Verification items for the finished model (mm, model axes). A direction names the side the tool comes from. Coordinates: 2 decimals unless noted, no trailing zeros. Write each loop counter-clockwise with the first axis right and the second up, starting at its lowest first coordinate (ties: lowest second). Pieces come first, ordered by that corner, then holes.
```python
from build123d import *

# Parameters (mm, degrees)
CUT_EXTRUDE1_REACH      = 26.41
CUT_EXTRUDE1_END_RADIUS = 1.524
SKETCH2_W               = 0.508
SKETCH2_H               = 0.889
CIRPATTERN1_COUNT       = 16
SKETCH3_R               = 3.556
SKETCH3_R_2             = 1.524
BOSS_EXTRUDE1_DEPTH     = 6.35
BOSS_EXTRUDE2_START     = 6.35
SKETCH4_R               = 19.05
SKETCH4_R_2             = 1.524
BOSS_EXTRUDE2_DEPTH     = 6.35
CUT_EXTRUDE2_REACH      = 51.396
SKETCH11_R              = 1.63195
CIRPATTERN2_COUNT       = 6
CHAMFER1_SIZE           = 3.048
CHAMFER1_SIZE2          = 5.279290861
SKETCH13_R              = 11.43
SKETCH13_R_2            = 6.54812
BOSS_EXTRUDE4_DEPTH     = 12.7
FILLET4_R               = 0.254
CHAMFER2_SIZE           = 0.851662
CHAMFER2_SIZE2          = 0.83947


with BuildPart() as part:
    # Sketch1 → Revolve2 (revolve)
    with BuildSketch(Plane.XY, mode=Mode.PRIVATE) as revolve2_sk:
        with BuildLine():
            Line((-1.524, 23.078774136), (-3.556, 23.078774136))
            Line((-3.556, 23.078774136), (-3.556, -2.067225864))
            ThreePointArc((-3.556, -2.067225864), (-2.514471714, -4.581697578), (0, -5.623225864))
            Line((0, -5.623225864), (0, -1.606607061))
            ThreePointArc((0, -1.606607061), (-0.720373994, -1.97463996), (-1.524, -2.067225864))
            Line((-1.524, -2.067225864), (-1.524, 23.078774136))
        make_face()
    revolve(revolve2_sk.sketch.rotate(Axis((0, 8.215698649, 0), (0, -1, 0)), 270), axis=Axis((0, 8.215698649, 0), (0, -1, 0)))

    # Cut-Extrude1: up to this cylinder (the profile starts outside it)
    cut_extrude1_end = Plane(origin=(0, -0.733726, 0), z_dir=(0, 1, 0)) * Cylinder(CUT_EXTRUDE1_END_RADIUS, 56.868, mode=Mode.PRIVATE)
    # Sketch2 → Cut-Extrude1 (cut, up to the surface)
    with BuildSketch(Plane.ZY.offset(3.556), mode=Mode.PRIVATE) as cut_extrude1_sk1:
        with Locations((0.000240101, -0.733725864)):
            Rectangle(SKETCH2_W, SKETCH2_H)
    cut_extrude1_tool1 = extrude(cut_extrude1_sk1.sketch, amount=-CUT_EXTRUDE1_REACH, mode=Mode.PRIVATE) - cut_extrude1_end
    cut_extrude1 = cut_extrude1_tool1.solids().sort_by_distance((-3.556, -0.733726, 0.00024))[0]
    add(cut_extrude1, mode=Mode.SUBTRACT)

    # CirPattern1: Cut-Extrude1 ×16 about axis
    cirpattern1_axis = Axis((0, 0, 0), (0, 1, 0))
    for i in range(1, CIRPATTERN1_COUNT):
        add(cut_extrude1.rotate(cirpattern1_axis, i * 360 / CIRPATTERN1_COUNT), mode=Mode.SUBTRACT)

    # Sketch3 → Boss-Extrude1 (add)
    with BuildSketch(Plane(origin=(0, 23.078774136, 0), x_dir=(-1, 0, 0), z_dir=(0, -1, 0))):
        with Locations(Location((0, 0, 0), (0, 0, 270))):
            Circle(SKETCH3_R)
        with Locations(Location((0, 0, 0), (0, 0, 270))):
            Circle(SKETCH3_R_2, mode=Mode.SUBTRACT)
    extrude(amount=-BOSS_EXTRUDE1_DEPTH)

    # Sketch4 → Boss-Extrude2 (add)
    with BuildSketch(Plane(origin=(0, 29.428774136, 0), x_dir=(1, 0, 0), z_dir=(0, 1, 0)).offset(BOSS_EXTRUDE2_START)):
        with Locations(Location((0, 0, 0), (0, 0, 270))):
            Circle(SKETCH4_R)
        with Locations(Location((0, 0, 0), (0, 0, 270))):
            Circle(SKETCH4_R_2, mode=Mode.SUBTRACT)
    extrude(amount=-BOSS_EXTRUDE2_DEPTH)

    # Sketch11 → Cut-Extrude2 (cut, up to next)
    with BuildSketch(Plane(origin=(0, 35.778774136, 0), x_dir=(1, 0, 0), z_dir=(0, 1, 0)), mode=Mode.PRIVATE) as cut_extrude2_sk1:
        with Locations(Location((0, -15.24, 0), (0, 0, 270))):
            Circle(SKETCH11_R)
    cut_extrude2_tool1 = extrude(cut_extrude2_sk1.sketch, amount=-CUT_EXTRUDE2_REACH, mode=Mode.PRIVATE) & part.part
    cut_extrude2 = cut_extrude2_tool1.solids().sort_by_distance((0, 35.778774, 15.24))[0]
    add(cut_extrude2, mode=Mode.SUBTRACT)

    # CirPattern2: Cut-Extrude2 ×6 about axis
    cirpattern2_axis = Axis((0, 0, 0), (0, 1, 0))
    for i in range(1, CIRPATTERN2_COUNT):
        add(cut_extrude2.rotate(cirpattern2_axis, i * 360 / CIRPATTERN2_COUNT), mode=Mode.SUBTRACT)

    # Chamfer1
    chamfer1_edges = [part.edges().sort_by_distance(p)[0] for p in [
        (0, 35.778774136, -1.524),
    ]]
    chamfer1_side = [part.faces().sort_by_distance(p)[0] for p in [
        (0, 35.778774136, -18.511184633),
    ]]
    chamfer(chamfer1_edges, length=CHAMFER1_SIZE, length2=CHAMFER1_SIZE2, reference=chamfer1_side[0])

    # Sketch13 → Boss-Extrude4 (add)
    with BuildSketch(Plane(origin=(0, 35.778774136, 0), x_dir=(1, 0, 0), z_dir=(0, 1, 0))):
        with Locations(Location((0, 0, 0), (0, 0, 270))):
            Circle(SKETCH13_R)
        with Locations(Location((0, 0, 0), (0, 0, 270))):
            Circle(SKETCH13_R_2, mode=Mode.SUBTRACT)
    extrude(amount=BOSS_EXTRUDE4_DEPTH)

    # Fillet4
    fillet4_edges = [part.edges().sort_by_distance(p)[0] for p in [
        (0, 35.778774136, -11.43),
    ]]
    fillet(fillet4_edges, radius=FILLET4_R)

    # Chamfer2
    chamfer2_edges = [part.edges().sort_by_distance(p)[0] for p in [
        (0, 48.478774136, -6.54812),
    ]]
    chamfer2_side = [part.faces().sort_by_distance(p)[0] for p in [
        (0, 48.478774136, -11.10671078),
    ]]
    chamfer(chamfer2_edges, length=CHAMFER2_SIZE, length2=CHAMFER2_SIZE2, reference=chamfer2_side[0])


solid = part.part
```
1. Sectioned sample at C-C, the plane y = 18. Record the boundary of the cut face in (x, z).
2. Material ranges on L1, parallel to X at y = 31, z = 7.62; L2, parallel to X at y = 27.5, z = 0; L3, parallel to Y at x = 12, z = -9.5, recorded low to high.
3. Draft check along Z on faces 4 (the cylindrical face through (11.333, 42.169, -1.488)), 5 (the flat face through (-1, -0.289, 2.3)), 6 (the flat face through (-4, 29.429, 0)). Enter one of: pulls with the +Z half, pulls with the -Z half, needs draft (parallel to the pull), parting line crosses it, or undercut.
4. Sectioned sample at B-B, the plane y = 43.5. Record the boundary of the cut face in (x, z).
5. Gauge pin test, flat ends, axial feed: P1, Ø1, axis at x = -2.5, z = 1, coming from the -Y side; P2, Ø0.6, axis at x = 0, z = -2, coming from the -Y side; P3, Ø0.9, axis at x = 1.5, z = 2, coming from the -Y side. Record the tip position at first contact, or that the pin passes through.
6. Sectioned sample at A-A, the plane z = -15.24. Record the boundary of the cut face in (x, y), and give its area (3 significant figures).
7. Tool access check on faces 1 (the flat face through (1.616, -0.74, 1.975)), 2 (the flat face through (-8, 35.779, -9)), 3 (the cylindrical face through (14.816, 32.648, -7.832)). Record the directions out of +Z, -Z, +X, -X, +Y, -Y that give a thin tool (end or side, any length) a straight path to the whole face; none if there is none.
Outcome:
1. outline: circle Ø7.11 at (0, 0); hole circle Ø3.05 at (0, 0)
2. L1: x = -17.46 to -14.83, -11.57 to 11.57, 14.83 to 17.46
2. L2: x = -3.56 to -1.52, 1.52 to 3.56
2. L3: y = 29.43 to 35.78
3. face 4: parting line crosses it
3. face 5: undercut
3. face 6: needs draft
4. outline: circle Ø22.86 at (0, 0); hole circle Ø13.1 at (0, 0)
5. P1: stops at y = -4.87
5. P2: stops at y = -5.19
5. P3: stops at y = -4.97
6. outline: (-11.43, 29.43) - (-1.63, 29.43) - (-1.63, 35.78) - (-11.43, 35.78) - close; (1.63, 29.43) - (11.43, 29.43) - (11.43, 35.78) - (1.63, 35.78) - close
6. area: 124 mm2
7. face 1: none
7. face 2: +Y
7. face 3: +Y, -Y
